CAD build for the part. Positions are in the model's coordinates, mm. A direction names the side the tool comes from. Round coordinates to 2 decimals unless told otherwise and drop trailing zeros. Write each loop counter-clockwise with the first axis right and the second up, starting at its lowest first coordinate (ties: lowest second). Pieces come first, ordered by that corner, then holes. Notation, with made-up numbers: (60, 28.25) - (109, 28.25) arc R22 cw to (109, 59.25) - close; hole circle Ø8 at (25.5, 23). An arc over 180 degrees is marked (long way). Answer in a Markdown table with one row per item.
```python
from build123d import *

# Parameters (mm, degrees)
SK_P01_STANDOFF_R                  = 2.5
P01_STANDOFF_DEPTH                 = 5
SK_P02_STANDOFF_R                  = 2.5
P02_STANDOFF_DEPTH                 = 5
P03_PERMAPROTOHALFSIZECARRIE_START = 5
SK_P03_PERMAPROTOHALFSIZECARRIE_W  = 81
SK_P03_PERMAPROTOHALFSIZECARRIE_H  = 51
P03_PERMAPROTOHALFSIZECARRIE_DEPTH = 1.6
P04_SOCKETROW_START                = 6.6
SK_P04_SOCKETROW_W                 = 63
SK_P04_SOCKETROW_H                 = 3
P04_SOCKETROW_DEPTH                = 8.5
P05_SOCKETROW_START                = 6.6
SK_P05_SOCKETROW_W                 = 63
SK_P05_SOCKETROW_H                 = 3
P05_SOCKETROW_DEPTH                = 8.5
P06_DEVKITC1_START                 = 15.1
SK_P06_DEVKITC1_W                  = 63
SK_P06_DEVKITC1_H                  = 25.4
P06_DEVKITC1_DEPTH                 = 1.6
P07_WROOM2MODULE_START             = 16.7
SK_P07_WROOM2MODULE_W              = 18
SK_P07_WROOM2MODULE_H              = 25.4
P07_WROOM2MODULE_DEPTH             = 3.2
P08_USBCX2_START                   = 16.7
SK_P08_USBCX2_W                    = 8
SK_P08_USBCX2_H                    = 21
P08_USBCX2_DEPTH                   = 3.3
P09_74LVC244_START                 = 6.6
SK_P09_74LVC244_W                  = 8
SK_P09_74LVC244_H                  = 27
P09_74LVC244_DEPTH                 = 5
P10_JSTXHHEADERSVERTICAL_START     = 6.6
SK_P10_JSTXHHEADERSVERTICAL_W      = 4
SK_P10_JSTXHHEADERSVERTICAL_H      = 47
P10_JSTXHHEADERSVERTICAL_DEPTH     = 6
P11_2X12BOXHEADERDECKSIGNALS_START = 6.6
SK_P11_2X12BOXHEADERDECKSIGNALS_W  = 40
SK_P11_2X12BOXHEADERDECKSIGNALS_H  = 9
P11_2X12BOXHEADERDECKSIGNALS_DEPTH = 9


with BuildPart() as part:
    # SK_P01_Standoff → P01_Standoff (new body)
    with BuildSketch(Plane(origin=(0, 0, 0), x_dir=(1, 0, 0), z_dir=(0, 1, 0))):
        with Locations(Location((-35.85, 0, 0), (0, 0, 270))):
            Circle(SK_P01_STANDOFF_R)
    extrude(amount=P01_STANDOFF_DEPTH)



with BuildPart() as body_2:
    # SK_P02_Standoff → P02_Standoff (new body)
    with BuildSketch(Plane(origin=(0, 0, 0), x_dir=(1, 0, 0), z_dir=(0, 1, 0))):
        with Locations(Location((37.85, 0, 0), (0, 0, 270))):
            Circle(SK_P02_STANDOFF_R)
    extrude(amount=P02_STANDOFF_DEPTH)


with BuildPart() as part_1:
    add(part.part)

    add(body_2.part)  # P03_PermaProtohalfsizecarrie merges body 2
    # SK_P03_PermaProtohalfsizecarrie → P03_PermaProtohalfsizecarrie (add)
    with BuildSketch(Plane(origin=(0, 0, 0), x_dir=(1, 0, 0), z_dir=(0, 1, 0)).offset(P03_PERMAPROTOHALFSIZECARRIE_START)):
        with Locations((1, 0)):
            Rectangle(SK_P03_PERMAPROTOHALFSIZECARRIE_W, SK_P03_PERMAPROTOHALFSIZECARRIE_H)
    extrude(amount=P03_PERMAPROTOHALFSIZECARRIE_DEPTH)

    # SK_P04_Socketrow → P04_Socketrow (add)
    with BuildSketch(Plane(origin=(0, 0, 0), x_dir=(1, 0, 0), z_dir=(0, 1, 0)).offset(P04_SOCKETROW_START)):
        with Locations((-9, 11.7)):
            Rectangle(SK_P04_SOCKETROW_W, SK_P04_SOCKETROW_H)
    extrude(amount=P04_SOCKETROW_DEPTH)

    # SK_P05_Socketrow → P05_Socketrow (add)
    with BuildSketch(Plane(origin=(0, 0, 0), x_dir=(1, 0, 0), z_dir=(0, 1, 0)).offset(P05_SOCKETROW_START)):
        with Locations((-9, -11.7)):
            Rectangle(SK_P05_SOCKETROW_W, SK_P05_SOCKETROW_H)
    extrude(amount=P05_SOCKETROW_DEPTH)

    # SK_P06_DevKitC1 → P06_DevKitC1 (add)
    with BuildSketch(Plane(origin=(0, 0, 0), x_dir=(1, 0, 0), z_dir=(0, 1, 0)).offset(P06_DEVKITC1_START)):
        with Locations((-9, 0)):
            Rectangle(SK_P06_DEVKITC1_W, SK_P06_DEVKITC1_H)
    extrude(amount=P06_DEVKITC1_DEPTH)

    # SK_P07_WROOM2module → P07_WROOM2module (add)
    with BuildSketch(Plane(origin=(0, 0, 0), x_dir=(1, 0, 0), z_dir=(0, 1, 0)).offset(P07_WROOM2MODULE_START)):
        with Locations((13.5, 0)):
            Rectangle(SK_P07_WROOM2MODULE_W, SK_P07_WROOM2MODULE_H)
    extrude(amount=P07_WROOM2MODULE_DEPTH)

    # SK_P08_USBCx2 → P08_USBCx2 (add)
    with BuildSketch(Plane(origin=(0, 0, 0), x_dir=(1, 0, 0), z_dir=(0, 1, 0)).offset(P08_USBCX2_START)):
        with Locations((-37.5, 0)):
            Rectangle(SK_P08_USBCX2_W, SK_P08_USBCX2_H)
    extrude(amount=P08_USBCX2_DEPTH)

    # SK_P09_74LVC244 → P09_74LVC244 (add)
    with BuildSketch(Plane(origin=(0, 0, 0), x_dir=(1, 0, 0), z_dir=(0, 1, 0)).offset(P09_74LVC244_START)):
        with Locations((29.5, 0)):
            Rectangle(SK_P09_74LVC244_W, SK_P09_74LVC244_H)
    extrude(amount=P09_74LVC244_DEPTH)

    # SK_P10_JSTXHheadersvertical → P10_JSTXHheadersvertical (add)
    with BuildSketch(Plane(origin=(0, 0, 0), x_dir=(1, 0, 0), z_dir=(0, 1, 0)).offset(P10_JSTXHHEADERSVERTICAL_START)):
        with Locations((38.5, 0)):
            Rectangle(SK_P10_JSTXHHEADERSVERTICAL_W, SK_P10_JSTXHHEADERSVERTICAL_H)
    extrude(amount=P10_JSTXHHEADERSVERTICAL_DEPTH)

    # SK_P11_2x12boxheaderdecksignals → P11_2x12boxheaderdecksignals (add)
    with BuildSketch(Plane(origin=(0, 0, 0), x_dir=(1, 0, 0), z_dir=(0, 1, 0)).offset(P11_2X12BOXHEADERDECKSIGNALS_START)):
        with Locations((-14.5, -20)):
            Rectangle(SK_P11_2X12BOXHEADERDECKSIGNALS_W, SK_P11_2X12BOXHEADERDECKSIGNALS_H)
    extrude(amount=P11_2X12BOXHEADERDECKSIGNALS_DEPTH)


solid = part_1.part
```
Q1. Pull direction Y, two halves, no side cores. Call faces 1 (the flat face through (-9, 11, -10.2)), 2 (the flat face through (-9, 11, 10.2)), 3 (the flat face through (29, 11.6, 0)), 4 (the flat face through (-41.5, 18, 0)): released by +Y, released by -Y, zero draft, split by the parting line, or undercut.
Computed:
| item | result |
|---|---|
| face 1 | undercut |
| face 2 | undercut |
| face 3 | released by +Y |
| face 4 | zero draft |
Q2. Saw through at B-B on x = -35.85. List the corners of the cut face in (y, z), then the cut area to 3 significant figures.
Computed:
| item | result |
|---|---|
| outline | (0, -2.5) - (5, -2.5) - (5, -25.5) - (6.6, -25.5) - (6.6, -13.2) - (15.1, -13.2) - (15.1, -12.7) - (16.7, -12.7) - (16.7, -10.5) - (20, -10.5) - (20, 10.5) - (16.7, 10.5) - (16.7, 12.7) - (15.1, 12.7) - (15.1, 13.2) - (6.6, 13.2) - (6.6, 25.5) - (5, 25.5) - (5, 2.5) - (0, 2.5) - close; hole (6.6, -10.2) - (15.1, -10.2) - (15.1, 10.2) - (6.6, 10.2) - close |
| area | 268 mm2 |
Q3. 3-axis set-ups, long thin cutter, end or side, ignore diameter. For faces 5 (the flat face through (38, 10, 23.5)), 6 (the flat face through (-38, 18, 10.5)), 7 (the flat face through (29, 9, -13.5)): which of +Z, -Z, +X, -X, +Y, -Y reach the whole face in a straight line?
Computed:
| item | result |
|---|---|
| face 5 | +Z, +X, +Y |
| face 6 | +Z, -X, +Y |
| face 7 | -Z, -X, +Y |
Q4. Saw through at D-D on z = -6.5. List the corners of the cut face in (x, y), then the cut area to 3 significant figures.
Computed:
| item | result |
|---|---|
| outline | (-41.5, 16.7) - (-40.5, 16.7) - (-40.5, 15.1) - (22.5, 15.1) - (22.5, 19.9) - (4.5, 19.9) - (4.5, 16.7) - (-33.5, 16.7) - (-33.5, 20) - (-41.5, 20) - close; (-39.5, 5) - (41.5, 5) - (41.5, 6.6) - (40.5, 6.6) - (40.5, 12.6) - (36.5, 12.6) - (36.5, 6.6) - (33.5, 6.6) - (33.5, 11.6) - (25.5, 11.6) - (25.5, 6.6) - (-39.5, 6.6) - close |
| area | 378 mm2 |
Q5. Drill centre lines: line 1 (Z direction, x = -16.5, y = 8.25); line 2 (Y direction, x = -13, z = -8); line 3 (X direction, y = 10, z = 20.5). Where is each one in solid material? Low to high.
Computed:
| item | result |
|---|---|
| line 1 | z = -13.2 to -10.2, 10.2 to 13.2, 15.5 to 24.5 |
| line 2 | y = 5 to 6.6, 15.1 to 16.7 |
| line 3 | x = -34.5 to 5.5, 36.5 to 40.5 |
Q6. Flat gauge pins, fed straight in: pin 1 (12 mm diameter, centred on y = 13, z = 19.5, fed in from +X); pin 2 (6.5 mm diameter, centred on y = 11, z = -7, fed in from -X); pin 3 (2 mm diameter, centred on x = 9.5, z = 1.5, fed in from -Y). Where does each tip first touch, or does it go through?
Computed:
| item | result |
|---|---|
| pin 1 | stops at x = 40.5 |
| pin 2 | stops at x = -40.5 |
| pin 3 | stops at y = 5 |
Q7. Saw through at C-C on x = 37.85. List the corners of the cut face in (y, z), then the cut area to 3 significant figures.
Computed:
| item | result |
|---|---|
| outline | (0, -2.5) - (5, -2.5) - (5, -25.5) - (6.6, -25.5) - (6.6, -23.5) - (12.6, -23.5) - (12.6, 23.5) - (6.6, 23.5) - (6.6, 25.5) - (5, 25.5) - (5, 2.5) - (0, 2.5) - close |
| area | 389 mm2 |
